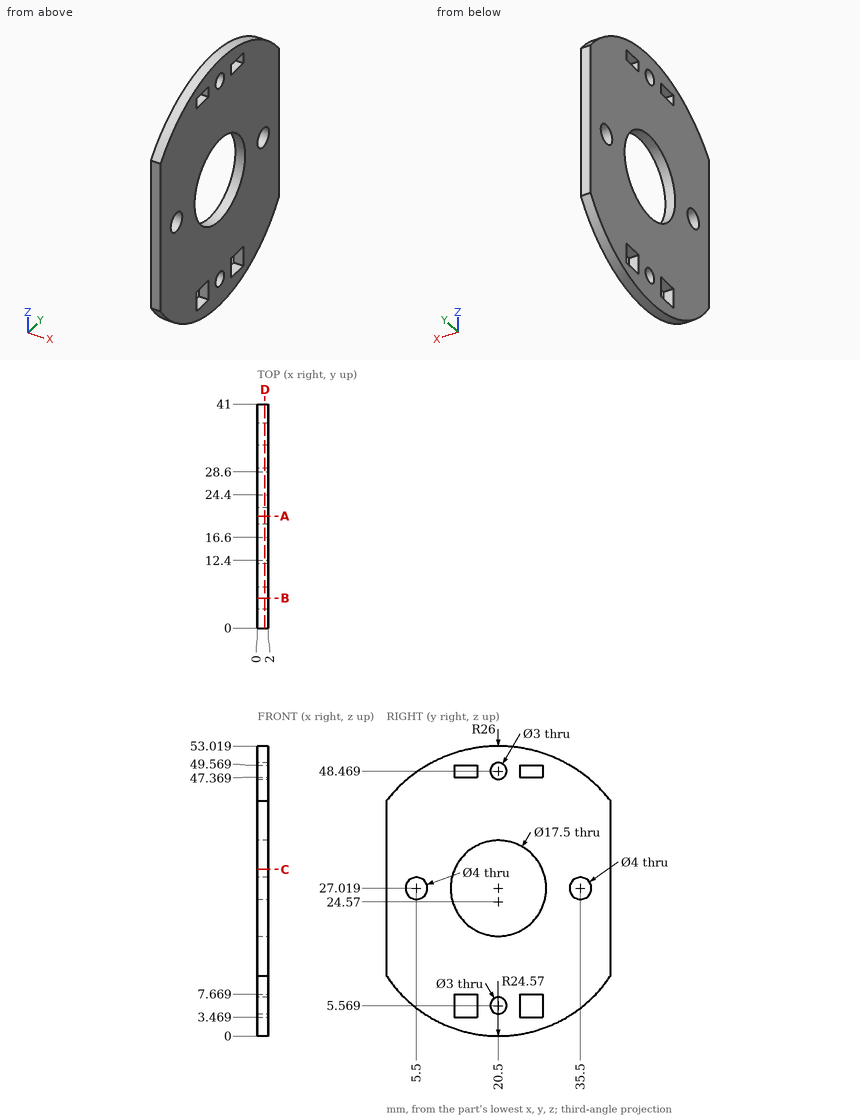
The drawing under review shows one solid part. Ordinate dimensions are in mm from its lowest x, y, z. Coordinates: 2 decimals unless noted, no trailing zeros. Write each loop counter-clockwise with the first axis right and the second up, starting at its lowest first coordinate (ties: lowest second). Pieces come first, ordered by that corner, then holes. Notation, with made-up numbers: M 2.5,20.5 L 52.5,20.5 A25 ccw 52.5,34.5 Z; hole C -8.5,-25.5 d1. An arc over 180 degrees is marked long. Answer as a JSON object with one key per item and string values.
Item 1: Add section C-C, the plane z = 30.5. Give the boundary of the cut face in (x, y).
Outcome:
{"outline": "M 0,0 L 2,0 L 2,12.47 L 0,12.47 Z; M 0,28.53 L 2,28.53 L 2,41 L 0,41 Z"}
Item 2: Add section A-A, the plane y = 20.5. Give the boundary of the cut face in (x, z).
Outcome:
{"outline": "M 0,0 L 2,0 L 2,4.07 L 0,4.07 Z; M 0,7.07 L 2,7.07 L 2,18.27 L 0,18.27 Z; M 0,35.77 L 2,35.77 L 2,46.97 L 0,46.97 Z; M 0,49.97 L 2,49.97 L 2,53.02 L 0,53.02 Z"}
Item 3: Add section D-D, the plane x = 1.35. State how many separate pieces and enclosed holes the cut face has, and give its area (3 significant figures).
Outcome:
{"separate pieces": "1", "enclosed holes": "9", "area": "1,580 mm²"}
Item 4: Wall thickness on probe 1 along Y at (x, z) = (1.3, 27); probe 2 along Y at (x, z) = (1.35, 27.5); probe 3 along Z at (x, y) = (1.6, 13.5): over which ranges is each line inside the solid? List them lowest first.
Outcome:
{"probe 1": "0 to 3.5, 7.5 to 11.75, 29.25 to 33.5, 37.5 to 41", "probe 2": "0 to 3.56, 7.44 to 11.76, 29.24 to 33.56, 37.44 to 41", "probe 3": "1.02 to 3.47, 7.67 to 21.77, 32.27 to 47.37, 49.57 to 52.06"}
Item 5: Insertion check: pin 1 Ø0.6 at (x, y) = (1, 15.5) entering from -Z; pin 2 Ø0.6 at (x, z) = (0.5, 49) entering from +Y; pin 3 Ø1 at (x, z) = (1, 5.5) entering from +Y. Each pin has a flat end and moves straight along its axis. Give the tip position at first contact, or say it passes through.
Outcome:
{"pin 1": "z = 0.45", "pin 2": "y = 34.85", "pin 3": "y = 36.59"}
Item 6: Add section B-B, the plane y = 5.5. Give the boundary of the cut face in (x, z) (1 decimal).
Outcome:
{"outline": "M 0,5.1 L 2,5.1 L 2,25 L 0,25 Z; M 0,29 L 2,29 L 2,48.3 L 0,48.3 Z"}
